For this review, take the finished solid that the model builds, in its own axes (mm). A direction names the side the tool comes from. Give positions to 0.01 mm unless a question says otherwise; leave off trailing zeros. Write each loop counter-clockwise with the first axis right and the second up, starting at its lowest first coordinate (ties: lowest second). Pieces come first, ordered by that corner, then holes. Notation, with made-up numbers: M 55.5,7.5 L 66.5,7.5 A29 ccw 66.5,43.5 Z; hole C -4,14 d3. An arc over 180 degrees is marked long. Write item = value, one per line.
```python
from build123d import *

# Parameters (mm, degrees)
F0_R     = 3.175
F1_DEPTH = 22.225
F3_R     = 5.5626
F4_DEPTH = 9.525
F6_DEPTH = 6.35


with BuildPart() as f1:
    # F0 (on Front) → F1 (new body)
    with BuildSketch(Plane.XZ):
        Circle(F0_R)
    extrude(amount=F1_DEPTH)

    # F3 (on face) → F4 (join)
    with BuildSketch(Plane.XZ.offset(22.225)):
        Circle(F3_R)
    extrude(amount=F4_DEPTH)

    # F5 (on face) → F6 (cut)
    with BuildSketch(Plane.XZ.offset(31.75)):
        Polygon((3.175, 1.833087), (0, 3.666174), (-3.175, 1.833087), (-3.175, -1.833087), (0, -3.666174), (3.175, -1.833087), align=None)
    extrude(amount=-F6_DEPTH, mode=Mode.SUBTRACT)


solid = f1.part
```
1. We need section A-A, the plane z = 0. Write out the cut boundary in (x, y) (3 decimals), then the cut area to 3 significant figures.
Responses:
outline = M -5.563,-31.75 L -3.175,-31.75 L -3.175,-25.4 L 3.175,-25.4 L 3.175,-31.75 L 5.563,-31.75 L 5.563,-22.225 L 3.175,-22.225 L 3.175,0 L -3.175,0 L -3.175,-22.225 L -5.563,-22.225 Z
area = 207 mm2
2. The part is to be moulded in two halves that separate along Z. For faces 4 (the face through (1.61, -28.619, 2.737)), 5 (the face through (2.4, -22.225, -2.4)), 6 (the face through (5.306, -26.921, 1.671)), say which applies: +Z half, -Z half, draft (parallel to the pull), parting line (faces both ways), or undercut.
Responses:
face_4 = undercut
face_5 = draft
face_6 = parting line
3. We need section D-D, the plane y = -23. Write out the cut boundary in (x, z), then the cut area to 3 significant figures.
Responses:
outline = C 0,0 d11.13
area = 97.2 mm2
4. We need section C-C, the plane y = -15.5. Write out the cut boundary in (x, z) (3 decimals).
Responses:
outline = C 0,0 d6.35
5. For line 1 along Y through (x, z) = (-1.75, 1.75); line 2 along Y through (x, z) = (0, -3.5) (3 decimals); line 3 along X through (y, z) = (-28, -0.5) (3 decimals), list the stretches that pass through material, from the lowest coordinate up. Write a range as from..to.
Responses:
line_1 = -25.4..0
line_2 = -25.4..-22.225
line_3 = -5.54..-3.175, 3.175..5.54
6. We need section B-B, the plane x = 1. Write out the cut boundary in (y, z) (3 decimals), then the cut area to 3 significant figures.
Responses:
outline = M -31.75,-5.472 L -22.225,-5.472 L -22.225,-3.013 L 0,-3.013 L 0,3.013 L -22.225,3.013 L -22.225,5.472 L -31.75,5.472 L -31.75,3.089 L -25.4,3.089 L -25.4,-3.089 L -31.75,-3.089 Z
area = 199 mm2
7. Insertion check: P1, Ø3, axis at y = -21.5, z = 3.5, coming from the -X side; P2, Ø5, axis at x = 1, y = -16.5, coming from the -Z side (3 decimals); P3, Ø3, axis at x = -3.5, y = -15.5, coming from the -Z side. Each pin has a flat end and moves straight along its axis. Give the tip position at first contact, or say it passes through.
Responses:
P1 = -5.11
P2 = -3.175
P3 = -2.47
8. Machinability: for faces 1 (the face through (-0.69, -10.96, -3.1)), 2 (the face through (0, 0, 0)), 3 (the face through (3.175, -29, 0)), which of the approach directions +Z, -Z, +X, -X, +Y, -Y give a long, thin tool a straight path to every point of the face, cutting with its end or side? Answer none if there is none.
Responses:
face_1 = +Y
face_2 = +Z, -Z, +X, -X, +Y
face_3 = -Y
